from build123d import *

# Parameters (mm, degrees)
SKETCH1_W           = 368.3
SKETCH1_H           = 457.2
BOSS_EXTRUDE1_DEPTH = 12.7
SKETCH2_W           = 38.1
SKETCH2_H           = 38.1
BOSS_EXTRUDE2_DEPTH = 25.4
SKETCH3_W           = 25.4
SKETCH3_H           = 25.4
CUT_EXTRUDE1_DEPTH  = 18.796
SKETCH4_W           = 12.7
SKETCH4_H           = 406.4
CUT_EXTRUDE2_DEPTH  = 12.7


with BuildPart() as part:
    # Sketch1 → Boss-Extrude1 (new body)
    with BuildSketch(Plane.XY):
        Rectangle(SKETCH1_W, SKETCH1_H)
    extrude(amount=BOSS_EXTRUDE1_DEPTH)

    # Sketch2 → Boss-Extrude2 (add)
    with BuildSketch(Plane.XY.offset(12.7)):
        with Locations((-165.1, 209.55)):
            Rectangle(SKETCH2_W, SKETCH2_H)
        with Locations((-165.1, -209.55)):
            Rectangle(SKETCH2_W, SKETCH2_H)
        with Locations((165.1, -209.55)):
            Rectangle(SKETCH2_W, SKETCH2_H)
        with Locations((165.1, 209.55)):
            Rectangle(SKETCH2_W, SKETCH2_H)
    extrude(amount=BOSS_EXTRUDE2_DEPTH)

    # Sketch3 → Cut-Extrude1 (cut)
    with BuildSketch(Plane.XY.offset(38.1)):
        with Locations((-165.1, 209.55)):
            Rectangle(SKETCH3_W, SKETCH3_H)
        with Locations((165.1, -209.55)):
            Rectangle(SKETCH3_W, SKETCH3_H)
        with Locations((165.1, 209.55)):
            Rectangle(SKETCH3_W, SKETCH3_H)
        with Locations((-165.1, -209.55)):
            Rectangle(SKETCH3_W, SKETCH3_H)
    extrude(amount=-CUT_EXTRUDE1_DEPTH, mode=Mode.SUBTRACT)

    # Sketch4 → Cut-Extrude2 (cut)
    with BuildSketch(Plane(origin=(0, 0, 0), x_dir=(-1, 0, 0), z_dir=(0, 0, -1))):
        with Locations((-171.45, 0)):
            Rectangle(SKETCH4_W, SKETCH4_H)
    extrude(amount=-CUT_EXTRUDE2_DEPTH, mode=Mode.SUBTRACT)


solid = part.part
Input: part model. Units: mm. Frame: model coordinates. A direction names the side the tool comes from. Round coordinates to 2 decimals unless told otherwise and drop trailing zeros. Order: outer loops, then holes, each group sorted by start corner. A loop starts at its lowest first (then second) coordinate and runs counter-clockwise, first axis right, second up. Notation, with made-up numbers: (1.5, -1) - (46.5, -1) arc R29 ccw to (46.5, 29) - close; hole circle Ø9 at (32.25, 20). An arc over 180 degrees is marked (long way). Answer as a JSON object with one key per item and string values. Group by question number.
(1) Cut plane C-C (z = 7). Return loops of the section in (x, y), then the cut area to 3 significant figures.
(2) Cut plane D-D (x = -73.5). Return loops of the section in (y, z).
(3) Material intervals for probe 1 along Y at (x, z) = (-157.5, 33.5); probe 2 along Y at (x, z) = (146.5, 30); probe 3 along X at (y, z) = (27.5, 5), sorted ascending. Write a range as from..to.
(4) Cut plane B-B (y = -88). Return loops of the section in (x, z), then the cut area to 3 significant figures.
(5) Pin query (flat end, axial travel): P1, Ø20.5, axis at x = -159, y = 213.5, coming from the +Z side; P2, Ø1.5, axis at y = -55.5, z = 14, coming from the -X side; P3, Ø12.5, axis at x = -170.5, y = -212.5, coming from the +Z side; P4, Ø10, axis at x = -73, y = -86.5, coming from the +Z side. Return the tip coordinate at first contact, or that it passes through.
(6) Reachability of faces 1 (the face through (-3, 3, 0)), 2 (the face through (-165, -190.5, 25)), 3 (the face through (152.4, -210, 29)), 4 (the face through (-146.05, 209, 25)), 5 (the face through (172, 197, 12.7)) from +Z, -Z, +X, -X, +Y, -Y: full face, straight path, thin tool, end or side. Return the list, or none.
(7) Draft query along Y for faces 6 (the face through (152.4, 209, 29)), 7 (the face through (165, -209, 19.304)), 8 (the face through (-3, 228.6, 10)), 9 (the face through (152, -209, 38.1)). Return one class per face: released by +Y, released by -Y, zero draft, split by the parting line, or undercut.
(8) Cut plane A-A (z = 30.5). Count the separate pieces of the cut face and the enclosed holes in it, then the cut area to 3 significant figures.
Here are the results:
{
 "1": {"outline": "(-184.15, -228.6) - (184.15, -228.6) - (184.15, 228.6) - (-184.15, 228.6) - close; hole (165.1, -203.2) - (177.8, -203.2) - (177.8, 203.2) - (165.1, 203.2) - close", "area": "163,000 mm^2"},
 "2": {"outline": "(-228.6, 0) - (228.6, 0) - (228.6, 12.7) - (-228.6, 12.7) - close"},
 "3": {"probe 1": "y = -228.6..-222.25, -196.85..-190.5, 190.5..196.85, 222.25..228.6", "probe 2": "y = -228.6..-190.5, 190.5..228.6", "probe 3": "x = -184.15..165.1, 177.8..184.15"},
 "4": {"outline": "(-184.15, 0) - (165.1, 0) - (165.1, 12.7) - (-184.15, 12.7) - close; (177.8, 0) - (184.15, 0) - (184.15, 12.7) - (177.8, 12.7) - close", "area": "4,520 mm^2"},
 "5": {"P1": "stops at z = 38.1", "P2": "passes through", "P3": "stops at z = 19.3", "P4": "stops at z = 12.7"},
 "6": {"face 1": "-Z, +X, -X, +Y, -Y", "face 2": "+Z, +X, -X", "face 3": "+Z", "face 4": "+Z, +Y, -Y", "face 5": "-Z"},
 "7": {"face 6": "undercut", "face 7": "undercut", "face 8": "released by +Y", "face 9": "zero draft"},
 "8": {"separate pieces": "4", "enclosed holes": "4", "area": "3,230 mm^2"}
}
